Geometry check sheet. Reference: the model listing, model coordinates, mm. A direction names the side the tool comes from. Give positions to 0.01 mm unless a question says otherwise; leave off trailing zeros. Write each loop counter-clockwise with the first axis right and the second up, starting at its lowest first coordinate (ties: lowest second). Pieces come first, ordered by that corner, then holes. Notation, with made-up numbers: (-33, -26) - (24, -26) arc R20 ccw to (24, -4) - close; hole circle Ø9 at (76, -31). An arc over 180 degrees is marked (long way). One line per question, with ' | ' between items. Start each with the question number.
Q1. Section check B-B on x = -17. Record the boundary of the cut face in (y, z).
Q2. Set-up check for faces 5 (the face through (-75.286, 9.903, 2.986)), 6 (the face through (-44, 41, 0)), 7 (the face through (-43.855, 60.219, 0.986)), 8 (the face through (23.55, 42.57, -16.63)): record each of +Z, -Z, +X, -X, +Y, -Y from which the full face is reachable in a straight line by a thin tool's end or side.
Q3. Section check A-A on y = 27. Record the boundary of the cut face in (x, z), and give its area (3 significant figures).
Q4. Release check for a two-part mould opening along X. For faces 1 (the face through (-68.348, 60.692, 0.986)), 2 (the face through (33.468, 41.804, -18.945)), 3 (the face through (21.94, 44.92, -18.41)), 4 (the face through (-82, 42, 4)) record: +X half, -X half, draft (parallel to the pull), parting line (faces both ways), or undercut.
Q5. Thickness scan on L1, parallel to Y at x = 28.5, z = -18.75; L2, parallel to Z at x = -20, y = 69; L3, parallel to Z at x = -72.5, y = 76.5. Record the ranges inside material, lowest first. Write a range as [from, to].
Q6. Gauge pin test, flat ends, axial feed: P1, Ø4, axis at y = 31, z = -3.5, coming from the -X side; P2, Ø3, axis at x = 0.5, y = 39, coming from the +Z side; P3, Ø0.6, axis at x = -58, z = 3, coming from the +Y side. Record the tip position at first contact, or that the pin passes through.
Q7. Section check C-C on y = 76.5. Record the boundary of the cut face in (x, z) (3 decimals), and give its area (3 significant figures).
```python
from build123d import *
from OCP.BRepFilletAPI import BRepFilletAPI_MakeFillet

# Parameters (mm, degrees)
BOSS_EXTRUDE1_DEPTH = 84
CUT_EXTRUDE2_START  = -1
CUT_EXTRUDE2_DEPTH  = 82
CUT_EXTRUDE3_START  = 4.4
CUT_EXTRUDE3_DEPTH  = 71.5
CUT_EXTRUDE4_DEPTH  = 84
FILLET2_R1          = 4
FILLET2_R2          = 0.5
BOSS_EXTRUDE3_DEPTH = 2
CUT_EXTRUDE5_DEPTH  = 4


with BuildPart() as part:
    # Sketch1 → Boss-Extrude1 (new body)
    with BuildSketch(Plane(origin=(0, 0, 0), x_dir=(1, 0, 0), z_dir=(0, 1, 0))):
        Polygon((0, 0), (38.302222156, 32.139380484), (42.801735424, 26.777069382), (8.506559603, -2), (-85.5, -2), (-85.5, 0), align=None)
    extrude(amount=BOSS_EXTRUDE1_DEPTH)

    # Sketch5 → Cut-Extrude2 (cut)
    with BuildSketch(Plane(origin=(0, 84, 0), x_dir=(1, 0, 0), z_dir=(0, 1, 0)).offset(CUT_EXTRUDE2_START)):
        Polygon((8.506559603, -2), (30.721848453, 16.640840681), (27.765025449, 20.164645119), (1.350229999, -2), align=None)
    extrude(amount=-CUT_EXTRUDE2_DEPTH, mode=Mode.SUBTRACT)

    # Sketch7 → Cut-Extrude3 (cut)
    with BuildSketch(Plane.XZ.offset(-83).offset(CUT_EXTRUDE3_START)):
        Polygon((4.285763267, -0.463204882), (-0.306577305, -5.936143258), (18.078489329, -21.363045891), (22.670829902, -15.890107515), align=None)
    extrude(amount=CUT_EXTRUDE3_DEPTH, mode=Mode.SUBTRACT)

    # Sketch8 → Cut-Extrude4 (cut)
    with BuildSketch(Plane.XZ):
        Polygon((42.801735424, -26.777069382), (37.108645825, -22), (26.218579037, -22), (38.302222156, -32.139380484), align=None)
    extrude(amount=-CUT_EXTRUDE4_DEPTH, mode=Mode.SUBTRACT)

    # Fillet2: one fillet with a radius per group of edges: ONE call of the kernel's fillet builder (fillet() takes one radius for all edges)
    fillet2_edges_1 = [part.edges().sort_by_distance(p)[0] for p in [
        (0, 42, 0),
        (-85.5, 84, 1),
        (26.218579037, 42, -22),
        (-85.5, 0, 1),
    ]]
    fillet2_edges_2 = [part.edges().sort_by_distance(p)[0] for p in [
        (11.935606321, 7.1, -10.015162862),
        (2.743073004, 42.85, -2.301711546),
        (21.128139639, 42.85, -17.728614178),
        (11.935606321, 78.6, -10.015162862),
    ]]
    fillet2 = BRepFilletAPI_MakeFillet(part.part.solid().wrapped)
    for e in fillet2_edges_1:
        fillet2.Add(FILLET2_R1, e.wrapped)
    for e in fillet2_edges_2:
        fillet2.Add(FILLET2_R2, e.wrapped)
    add(Compound.cast(fillet2.Shape()), mode=Mode.REPLACE)

    # Sketch10 → Boss-Extrude3 (add)
    with BuildSketch(Plane.XY.offset(2)):
        with BuildLine():
            Line((-55.5, 79.8), (-55.5, 81.8))
            Line((-55.5, 81.8), (-63.3, 81.8))
            ThreePointArc((-63.3, 81.8), (-77.442135624, 75.942135624), (-83.3, 61.8))
            Line((-83.3, 61.8), (-83.3, 22.2))
            ThreePointArc((-83.3, 22.2), (-77.442135624, 8.057864376), (-63.3, 2.2))
            Line((-63.3, 2.2), (-55.5, 2.2))
            Line((-55.5, 2.2), (-55.5, 4.2))
            Line((-55.5, 4.2), (-61.3, 4.2))
            ThreePointArc((-61.3, 4.2), (-75.442135624, 10.057864376), (-81.3, 24.2))
            Line((-81.3, 24.2), (-81.3, 59.8))
            ThreePointArc((-81.3, 59.8), (-75.442135624, 73.942135624), (-61.3, 79.8))
            Line((-61.3, 79.8), (-55.5, 79.8))
        make_face()
    extrude(amount=BOSS_EXTRUDE3_DEPTH)

    # Sketch11 → Cut-Extrude5 (cut)
    with BuildSketch(Plane(origin=(0, 0, 0), x_dir=(-1, 0, 0), z_dir=(0, 0, -1))):
        with BuildLine():
            ThreePointArc((49.386884986, 71.331085509), (43.350190066, 60.385387064), (49.811095522, 49.684606686))
            Line((49.811095522, 49.684606686), (50.052563318, 50.122434624))
            ThreePointArc((50.052563318, 50.122434624), (43.850094081, 60.395183787), (49.645321205, 70.903054294))
            Line((49.645321205, 70.903054294), (49.386884986, 71.331085509))
        make_face()
        with BuildLine():
            Line((62.050259679, 50.357555968), (62.308695897, 49.929524753))
            ThreePointArc((62.308695897, 49.929524753), (68.345390817, 60.875223198), (61.884485362, 71.576003576))
            Line((61.884485362, 71.576003576), (61.643017565, 71.138175638))
            ThreePointArc((61.643017565, 71.138175638), (67.845486802, 60.865426475), (62.050259679, 50.357555968))
        make_face()
        with BuildLine():
            ThreePointArc((50.679066077, 69.190929433), (45.849710141, 60.434370678), (51.018434506, 51.873746375))
            Line((51.018434506, 51.873746375), (51.259902302, 52.311574313))
            ThreePointArc((51.259902302, 52.311574313), (46.349614156, 60.4441674), (50.937502296, 68.762898218))
            Line((50.937502296, 68.762898218), (50.679066077, 69.190929433))
        make_face()
        with BuildLine():
            Line((60.758078588, 52.497712044), (61.016514806, 52.069680829))
            ThreePointArc((61.016514806, 52.069680829), (65.845870742, 60.826239584), (60.677146378, 69.386863887))
            Line((60.677146378, 69.386863887), (60.435678581, 68.949035949))
            ThreePointArc((60.435678581, 68.949035949), (65.345966727, 60.816442862), (60.758078588, 52.497712044))
        make_face()
        with BuildLine():
            ThreePointArc((51.971247168, 67.050773358), (48.349230216, 60.483354291), (52.22577349, 54.062886064))
            Line((52.22577349, 54.062886064), (52.467241286, 54.500714002))
            ThreePointArc((52.467241286, 54.500714002), (48.849134231, 60.493151014), (52.229683387, 66.622742143))
            Line((52.229683387, 66.622742143), (51.971247168, 67.050773358))
        make_face()
        with BuildLine():
            Line((59.465897497, 54.637868119), (59.724333715, 54.209836904))
            ThreePointArc((59.724333715, 54.209836904), (63.346350667, 60.777255971), (59.469807394, 67.197724198))
            Line((59.469807394, 67.197724198), (59.228339597, 66.75989626))
            ThreePointArc((59.228339597, 66.75989626), (62.846446652, 60.767459248), (59.465897497, 54.637868119))
        make_face()
        with BuildLine():
            ThreePointArc((53.26342826, 64.910617282), (50.848750292, 60.532337904), (53.433112474, 56.252025753))
            Line((53.433112474, 56.252025753), (53.67458027, 56.689853691))
            ThreePointArc((53.67458027, 56.689853691), (51.348654307, 60.542134627), (53.521864478, 64.482586067))
            Line((53.521864478, 64.482586067), (53.26342826, 64.910617282))
        make_face()
        with BuildLine():
            Line((58.173716406, 56.778024195), (58.432152624, 56.34999298))
            ThreePointArc((58.432152624, 56.34999298), (60.846830592, 60.728272358), (58.26246841, 65.008584509))
            Line((58.26246841, 65.008584509), (58.021000613, 64.570756571))
            ThreePointArc((58.021000613, 64.570756571), (60.346926577, 60.718475635), (58.173716406, 56.778024195))
        make_face()
        with BuildLine():
            ThreePointArc((54.555609351, 62.770461207), (53.348270367, 60.581321518), (54.640451458, 58.441165442))
            Line((54.640451458, 58.441165442), (54.881919254, 58.87899338))
            ThreePointArc((54.881919254, 58.87899338), (53.848174382, 60.59111824), (54.814045569, 62.342429991))
            Line((54.814045569, 62.342429991), (54.555609351, 62.770461207))
        make_face()
        with BuildLine():
            Line((56.881535314, 58.91818027), (57.139971533, 58.490149055))
            ThreePointArc((57.139971533, 58.490149055), (58.347310517, 60.679288744), (57.055129426, 62.81944482))
            Line((57.055129426, 62.81944482), (56.813661629, 62.381616882))
            ThreePointArc((56.813661629, 62.381616882), (57.847406502, 60.669492022), (56.881535314, 58.91818027))
        make_face()
    extrude(amount=-CUT_EXTRUDE5_DEPTH, mode=Mode.SUBTRACT)


solid = part.part
```
Working result:
1) outline: (0, 0) - (84, 0) - (84, 2) - (0, 2) - close
2) face 5: +Z, +X | face 6: -Z, -X, +Y, -Y | face 7: +Z, -Z | face 8: +Z
3) outline: (-85.5, 0) - (-1.46, 0) arc R4 cw to (1.12, -0.94) - (2.36, -1.98) arc R0.5 ccw to (3.06, -1.92) - (4.29, -0.46) - (1.35, 2) - (-81.3, 2) - (-81.3, 4) - (-83.3, 4) - (-83.3, 2) - (-85.5, 2) - close; (21.45, -17.35) arc R0.5 ccw to (21.51, -18.05) - (25.1, -21.06) arc R4 ccw to (27.67, -22) - (37.11, -22) - (30.72, -16.64) - (27.77, -20.16) - (22.67, -15.89) - close | area: 230 mm2
4) face 1: undercut | face 2: +X half | face 3: -X half | face 4: draft
5) L1: y = [0, 1], [83, 84] | L2: z = [0, 2] | L3: z = [0, 4]
6) P1: stops at x = 1.79 | P2: stops at z = 2 | P3: stops at y = 81.8
7) outline: (-85.5, 0) - (-1.456, 0) arc R4 cw to (1.115, -0.936) - (2.36, -1.98) arc R0.5 ccw to (3.064, -1.919) - (4.286, -0.463) - (1.35, 2) - (-72.305, 2) - (-72.305, 4) - (-76.861, 4) - (-76.861, 2) - (-85.5, 2) - close; (21.45, -17.346) arc R0.5 ccw to (21.511, -18.05) - (25.103, -21.064) arc R4 ccw to (27.674, -22) - (37.109, -22) - (30.722, -16.641) - (27.765, -20.165) - (22.671, -15.89) - close | area: 235 mm2
